Source: three-view drawing plus pictorial views. Frame: mm from the lowest corner of the part. A direction names the side the tool comes from. Coordinates: 2 decimals unless noted, no trailing zeros. Write each loop counter-clockwise with the first axis right and the second up, starting at its lowest first coordinate (ties: lowest second). Pieces come first, ordered by that corner, then holes. Notation, with made-up numbers: (-11, -39.5) -> (10, -39.5) arc R18 ccw to (10, -33.5) -> close; hole circle Ø5 at (23, 76). An arc over 180 degrees is marked (long way). One line per item, written item: value. Start each with the question number.
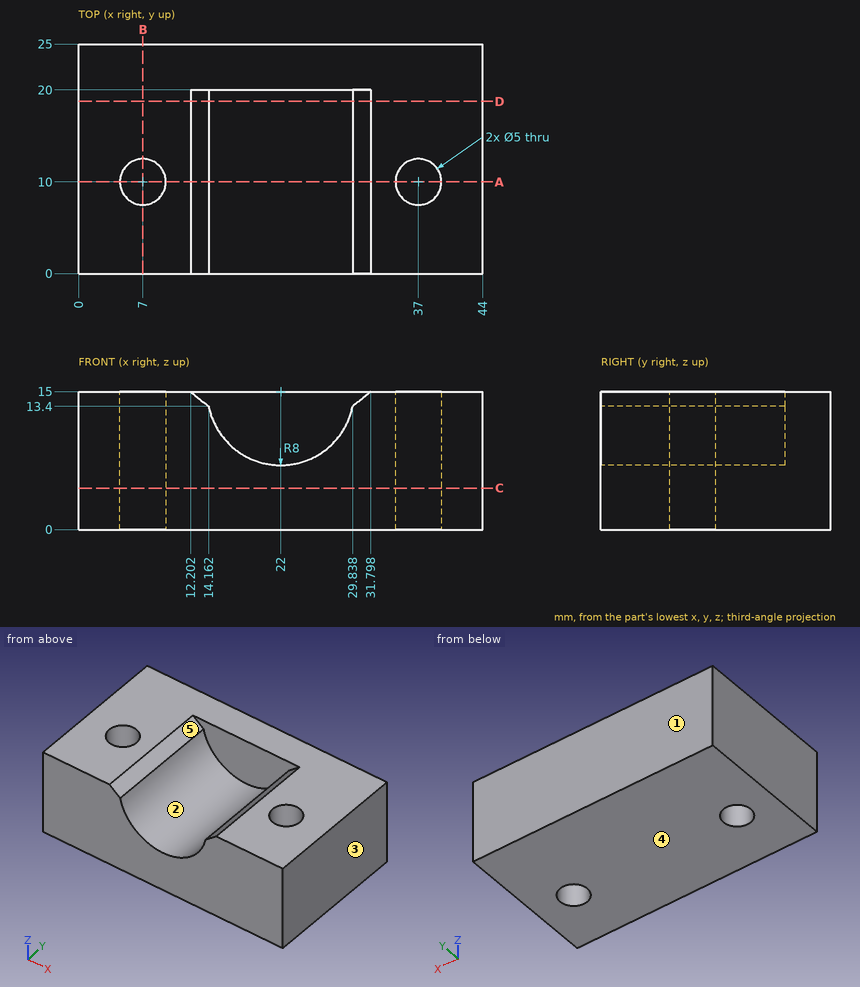
Q1. First-contact query: P1, Ø2.5, axis at x = 25.5, z = 12.5, coming from the -Y side. Flat tip, straight axial feed; report the tip coordinate or a pass-through.
Q2. Draft query along X for the marked faces 3, 4 and 5. Return one class per face: pulls with the +X half, pulls with the -X half, needs draft (parallel to the pull), parting line crosses it, or undercut.
Q3. Cut plane A-A on y = 10. Output: boundary loops of the cut face in (x, z).
Q4. Cut plane C-C on z = 4.5. Output: boundary loops of the cut face in (x, y), and give its area (3 significant figures).
Q5. Access query for the marked faces 1 and 2. Directions: +Z, -Z, +X, -X, +Y, -Y. A direction counts if a zero-diameter tool reaches every point of the face in a straight line with its end or side. Return the directions, or none.
Q6. Cut plane D-D on y = 18.75. Output: boundary loops of the cut face in (x, z), and give its area (3 significant figures).
Q7. Cut plane B-B on x = 7. Output: boundary loops of the cut face in (y, z).
Q8. Line query: L1, parallel to Y at x = 37, z = 4.5; L2, parallel to X at y = 7.75, z = 6.25; L3, parallel to Y at x = 23, z = 7.5. Output: solid intervals per line, ascending. Write a range as from..to.
Solution:
1. P1: y = 20
2. face 3: pulls with the +X half
2. face 4: needs draft
2. face 5: undercut
3. outline: (0, 0) -> (4.5, 0) -> (4.5, 15) -> (0, 15) -> close; (9.5, 0) -> (34.5, 0) -> (34.5, 15) -> (31.8, 15) -> (29.84, 13.4) arc R8 cw to (14.16, 13.4) -> (12.2, 15) -> (9.5, 15) -> close; (39.5, 0) -> (44, 0) -> (44, 15) -> (39.5, 15) -> close
4. outline: (0, 0) -> (44, 0) -> (44, 25) -> (0, 25) -> close; hole circle Ø5 at (7, 10); hole circle Ø5 at (37, 10)
4. area: 1,060 mm²
5. face 1: +Z, -Z, +X, -X, +Y
5. face 2: +Z, -Y
6. outline: (0, 0) -> (44, 0) -> (44, 15) -> (31.8, 15) -> (29.84, 13.4) arc R8 cw to (14.16, 13.4) -> (12.2, 15) -> (0, 15) -> close
6. area: 557 mm²
7. outline: (0, 0) -> (7.5, 0) -> (7.5, 15) -> (0, 15) -> close; (12.5, 0) -> (25, 0) -> (25, 15) -> (12.5, 15) -> close
8. L1: 0..7.5, 12.5..25
8. L2: 0..5.91, 8.09..35.91, 38.09..44
8. L3: 20..25
